Geometry: final body of the model. Coordinates: model frame, mm. Face numbers are marked on the shaded views. A direction names the side the tool comes from. Round coordinates to 2 decimals unless told otherwise and drop trailing zeros. Order: outer loops, then holes, each group sorted by start corner. A loop starts at its lowest first (then second) coordinate and runs counter-clockwise, first axis right, second up. Notation, with made-up numbers: (64, 85.25) -> (73, 85.25) arc R19 ccw to (73, 96.25) -> close; hole circle Ø7 at (-6, 11.25). An arc over 180 degrees is marked (long way). Put each result on its own line as item: value.
```python
from build123d import *

# Parameters (mm, degrees)
CROQUIS1_R              = 7.9375
SALIENTE_EXTRUIR1_DEPTH = 160
SALIENTE_EXTRUIR2_DEPTH = 10
CROQUIS3_R              = 34.921607703
CROQUIS3_R_2            = 12
CORTAR_EXTRUIR1_DEPTH   = 6
CORTAR_EXTRUIR1_DRAFT   = -46


with BuildPart() as part:
    # Croquis1 → Saliente-Extruir1 (new body)
    with BuildSketch(Plane.XY):
        Circle(CROQUIS1_R)
    extrude(amount=SALIENTE_EXTRUIR1_DEPTH)

    # Croquis2 → Saliente-Extruir2 (add)
    with BuildSketch(Plane.XY.offset(160)):
        Polygon((13.856406461, 0), (6.92820323, 12), (-6.92820323, 12), (-13.856406461, 0), (-6.92820323, -12), (6.92820323, -12), align=None)
    extrude(amount=SALIENTE_EXTRUIR2_DEPTH)


with BuildPart() as cortar_extruir1_tool:
    # Croquis3 → Cortar-Extruir1 (with draft: the straight prism first)
    with BuildSketch(Plane.XY.offset(170)):
        Circle(CROQUIS3_R)
        Circle(CROQUIS3_R_2, mode=Mode.SUBTRACT)
    extrude(amount=-CORTAR_EXTRUIR1_DEPTH)
    # Cortar-Extruir1: the draft: its side faces are tilted about the plane it starts from
    cortar_extruir1_sides = [cortar_extruir1_tool.faces().sort_by_distance(p)[0] for p in [
        (-34.921607703, 0, 167),
        (-12, 0, 167),
    ]]
    draft(cortar_extruir1_sides, Plane.XY.offset(170), CORTAR_EXTRUIR1_DRAFT)


with BuildPart() as part_1:
    add(part.part)

    # Cortar-Extruir1: cut by cortar_extruir1_tool
    add(cortar_extruir1_tool.part, mode=Mode.SUBTRACT)


solid = part_1.part
```
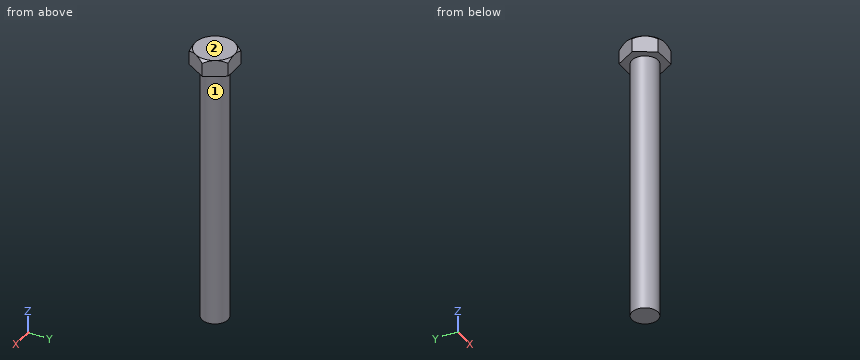
1. Set-up query: the marked faces 1 and 2. Return all of +Z, -Z, +X, -X, +Y, -Y with unobstructed straight access to the full face (end or side cutting, diameter ignored); none if empty.
Ans:
face 1: -Z
face 2: +Z, +X, -X, +Y, -Y
2. Cut plane A-A on z = 146. Return loops of the section in (x, y) (1 decimal).
Ans:
outline: circle Ø15.9 at (0, 0)
3. Material intervals for probe 1 along X at (y, z) = (0.5, 153.5); probe 2 along Z at (x, y) = (-10, 2.5); probe 3 along X at (y, z) = (5, 159), sorted ascending.
Ans:
probe 1: -7.92 to 7.92
probe 2: 160 to 170
probe 3: -6.16 to 6.16
4. Contact query for flat-ended pins moving along their axis: P1, Ø2, axis at x = -3.5, z = 117, coming from the -Y side; P2, Ø5, axis at x = 4, z = 42, coming from the +Y side; P3, Ø4, axis at y = -2.5, z = 145.5, coming from the -X side. Output: stop coordinate, or through.
Ans:
P1: y = -7.53
P2: y = 7.79
P3: x = -7.92
